Autodesk Inventor part; units mm, degrees
ref_plane "dia1_XY" through (-3.175, 3.9624, 0) normal (1, 0, 0) x (0, 0, -1)
ref_plane "dia1_YZ" through (-3.175, 3.9624, 0) normal (0, 0, -1) x (0, 1, 0)
ref_plane "dia1_ZX" through (-3.175, 3.9624, 0) normal (0, 1, 0) x (1, 0, 0)
sketch "Sketch_1" plane through (0, 0, 0) normal (0, 0, 1) x (1, 0, 0)
  line L0 (164.973, 0) -> (-3.175, 0)
  line L1 (-3.175, 0) -> (-3.175, 3.9624)
  line L2 (-3.175, 3.9624) -> (142.875, 3.9624)
  line L3 (142.875, 3.9624) -> (142.875, 13.5572)
  line L4 (142.875, 13.5572) -> (164.973, 13.5572)
  line L5 (164.973, 13.5572) -> (164.973, 0)
  line L6 (164.973, 0) -> (-3.175, 0)
revolve "Revolution1" add sketch "Sketch_1" angle 360 about axis through (164.973, 0, 0) along (1, 0, 0)
sketch "Sketch_3" plane through (0, 0, 0) normal (0, 0, 1) x (1, 0, 0)
  line L0 (-3.175, 0) -> (-15.875, 0)
  line L1 (-15.875, 0) -> (-15.875, 3.3388)
  line L2 (-15.875, 3.3388) -> (-15.2451, 3.9688)
  line L3 (-15.2451, 3.9688) -> (-3.175, 3.9688)
  line L4 (-3.175, 3.9688) -> (-3.175, 0)
  line L5 (-3.175, 0) -> (-15.875, 0)
revolve "Revolution2" add sketch "Sketch_3" angle 360 about axis through (-3.175, 0, 0) along (1, 0, 0)
thread "Thread1"
sketch "Sketch_10" plane through (-3.175, 0, 0) normal (1, 0, 0) x (0, 0, -1)
  line L0 (-7.9248, -7.9248) -> (7.9248, -7.9248)
  line L1 (7.9248, -7.9248) -> (7.9248, 7.9248)
  line L2 (7.9248, 7.9248) -> (-7.9248, 7.9248)
  line L3 (-7.9248, 7.9248) -> (-7.9248, -7.9248)
  line L4 (-3.175, -3.9624) -> (3.175, -3.9624)
  line L5 (3.175, -3.9624) -> (3.175, 3.9624)
  line L6 (3.175, 3.9624) -> (-3.175, 3.9624)
  line L7 (-3.175, 3.9624) -> (-3.175, -3.9624)
extrude "Extrusion1" cut sketch "Sketch_10" along normal blind 3.175
ref_plane "dia1_XY" through (-3.175, 3.9624, 0) normal (1, 0, 0) x (0, 0, -1)
ref_plane "dia1_YZ" through (-3.175, 3.9624, 0) normal (0, 0, -1) x (0, 1, 0)
ref_plane "dia1_ZX" through (-3.175, 3.9624, 0) normal (0, 1, 0) x (1, 0, 0)
ref_plane "dia12_XY" through (0, 0, 14.1351) normal (1, 0, 0) x (0, 0, -1)
ref_plane "dia12_YZ" through (0, 0, 14.1351) normal (0, 0, -1) x (0, 1, 0)
ref_plane "dia12_ZX" through (0, 0, 14.1351) normal (0, 1, 0) x (1, 0, 0)
ref_plane "dia2_XY" through (-3.175, -3.9624, 0) normal (1, 0, 0) x (0, 0, -1)
ref_plane "dia2_YZ" through (-3.175, -3.9624, 0) normal (0, 0, -1) x (0, 1, 0)
ref_plane "dia2_ZX" through (-3.175, -3.9624, 0) normal (0, 1, 0) x (1, 0, 0)
ref_plane "dia22_XY" through (0, 0, -14.1351) normal (1, 0, 0) x (0, 0, -1)
ref_plane "dia22_YZ" through (0, 0, -14.1351) normal (0, 0, -1) x (0, 1, 0)
ref_plane "dia22_ZX" through (0, 0, -14.1351) normal (0, 1, 0) x (1, 0, 0)
ref_plane "rl1_XY" through (-15.875, 0, 0) normal (1, 0, 0) x (0, 0, -1)
ref_plane "rl1_YZ" through (-15.875, 0, 0) normal (0, 0, -1) x (0, 1, 0)
ref_plane "rl1_ZX" through (-15.875, 0, 0) normal (0, 1, 0) x (1, 0, 0)
ref_plane "rl2_XY" through (-3.175, 0, 0) normal (1, 0, 0) x (0, 0, -1)
ref_plane "rl2_YZ" through (-3.175, 0, 0) normal (0, 0, -1) x (0, 1, 0)
ref_plane "rl2_ZX" through (-3.175, 0, 0) normal (0, 1, 0) x (1, 0, 0)
ref_plane "rod_cp_XY" through (0, 0, 0) normal (1, 0, 0) x (0, 0, -1)
ref_plane "rod_cp_YZ" through (0, 0, 0) normal (0, 0, -1) x (0, 1, 0)
ref_plane "rod_cp_ZX" through (0, 0, 0) normal (0, 1, 0) x (1, 0, 0)
ref_plane "thd1_XY" through (-15.875, 3.9688, 0) normal (1, 0, 0) x (0, 0, -1)
ref_plane "thd1_YZ" through (-15.875, 3.9688, 0) normal (0, 0, -1) x (0, 1, 0)
ref_plane "thd1_ZX" through (-15.875, 3.9688, 0) normal (0, 1, 0) x (1, 0, 0)
ref_plane "thd2_XY" through (-15.875, -3.9688, 0) normal (1, 0, 0) x (0, 0, -1)
ref_plane "thd2_YZ" through (-15.875, -3.9688, 0) normal (0, 0, -1) x (0, 1, 0)
ref_plane "thd2_ZX" through (-15.875, -3.9688, 0) normal (0, 1, 0) x (1, 0, 0)
ref_plane "to_rod_clevis_XY" through (-20.701, 0, 0) normal (1, 0, 0) x (0, 0, -1)
ref_plane "to_rod_clevis_YZ" through (-20.701, 0, 0) normal (0, 0, -1) x (0, 1, 0)
ref_plane "to_rod_clevis_ZX" through (-20.701, 0, 0) normal (0, 1, 0) x (1, 0, 0)
ref_plane "wf1_XY" through (-3.175, 0, 0) normal (1, 0, 0) x (0, 0, -1)
ref_plane "wf1_YZ" through (-3.175, 0, 0) normal (0, 0, -1) x (0, 1, 0)
ref_plane "wf1_ZX" through (-3.175, 0, 0) normal (0, 1, 0) x (1, 0, 0)
ref_plane "wf2_XY" through (0, 0, 0) normal (1, 0, 0) x (0, 0, -1)
ref_plane "wf2_YZ" through (0, 0, 0) normal (0, 0, -1) x (0, 1, 0)
ref_plane "wf2_ZX" through (0, 0, 0) normal (0, 1, 0) x (1, 0, 0)
ref_plane "wfw1_XY" through (-3.175, 0, -3.175) normal (0, 1, 0) x (1, 0, 0)
ref_plane "wfw1_YZ" through (-3.175, 0, -3.175) normal (1, 0, 0) x (0, 0, -1)
ref_plane "wfw1_ZX" through (-3.175, 0, -3.175) normal (0, 0, -1) x (0, 1, 0)
ref_plane "wfw2_XY" through (-3.175, 0, 3.175) normal (0, 1, 0) x (1, 0, 0)
ref_plane "wfw2_YZ" through (-3.175, 0, 3.175) normal (1, 0, 0) x (0, 0, -1)
ref_plane "wfw2_ZX" through (-3.175, 0, 3.175) normal (0, 0, -1) x (0, 1, 0)
properties part number "SR-094-D0_rod"
The model under review builds one solid part; all positions refer to its coordinate system, in mm. A direction names the side the tool comes from. Give positions to 0.01 mm unless a question says otherwise; leave off trailing zeros. Write each loop counter-clockwise with the first axis right and the second up, starting at its lowest first coordinate (ties: lowest second). Pieces come first, ordered by that corner, then holes. Notation, with made-up numbers: (0, 16.25) - (59, 16.25) arc R22 cw to (59, 29.25) - close; hole circle Ø2 at (23.5, -31.75). An arc over 180 degrees is marked (long way). Answer in a Markdown table with one row per item. Add a question column.
1. We need section A-A on z = 0. Write out the cut boundary in (x, y) (3 decimals).
2. We need section D-D on y = 9.75. Write out the cut boundary in (x, z) (3 decimals).
3. Tool access review of faces 5 (the flat face through (164.973, 0, 0)), 6 (the cylindrical face through (-9.126, 3.666, -1.52)): name each direction out of +Z, -Z, +X, -X, +Y, -Y from which nothing blocks a thin tool from reaching the whole face with its end or side.
4. Wall thickness on line 1 along X through (y, z) = (-0.5, -4.5) (3 decimals); line 2 along Z through (x, y) = (5, 0.25); line 3 along X through (y, z) = (3, -1.75): over which ranges is each line inside the solid? List them lowest first. Write a range as [from, to].
5. We need section C-C on x = 27. Write out the cut boundary in (y, z).
6. Draft analysis for pull direction X (two halves, no side actions). For faces 1 (the flat face through (-15.875, 0, 0)), 2 (the flat face through (-2, 0, -3.175)), 3 (the flat face through (-2, 0, 3.175)), 4 (the cylindrical face through (154.08, 12.93, 4.07)), state which applies: +X half, -X half, draft (parallel to the pull), parting line (faces both ways), or undercut.
7. Insertion check: P1, Ø2.5, axis at x = -2, y = 0.5, coming from the -Z side; P2, Ø5, axis at y = 10.5, z = -10.5, coming from the -X side (3 decimals); P3, Ø3.5, axis at x = -1, y = -0.5, coming from the +Z side. Each pin has a flat end and moves straight along its axis. Give the tip position at first contact, or say it passes through.
8. We need section B-B on y = 0. Write out the cut boundary in (x, z) (3 decimals), then the cut area to 3 significant figures.
Ans:
| question | item | result |
|---|---|---|
| 1 | outline | (-15.875, -3.339) - (-15.245, -3.969) - (-3.175, -3.969) - (-3.175, -3.962) - (142.875, -3.962) - (142.875, -13.557) - (164.973, -13.557) - (164.973, 13.557) - (142.875, 13.557) - (142.875, 3.962) - (-3.175, 3.962) - (-3.175, 3.969) - (-15.245, 3.969) - (-15.875, 3.339) - close |
| 2 | outline | (142.875, -9.42) - (164.973, -9.42) - (164.973, 9.42) - (142.875, 9.42) - close |
| 3 | face 5 | +Z, -Z, +X, +Y, -Y |
| 3 | face 6 | -X |
| 4 | line 1 | x = [142.875, 164.973] |
| 4 | line 2 | z = [-3.95, 3.95] |
| 4 | line 3 | x = [-15.74, 164.97] |
| 5 | outline | circle Ø7.92 at (0, 0) |
| 6 | face 1 | -X half |
| 6 | face 2 | undercut |
| 6 | face 3 | undercut |
| 6 | face 4 | draft |
| 7 | P1 | stops at z = -3.97 |
| 7 | P2 | stops at x = 142.875 |
| 7 | P3 | stops at z = 3.96 |
| 8 | outline | (-15.875, -3.339) - (-15.245, -3.969) - (-3.175, -3.969) - (-3.175, -3.175) - (0, -3.175) - (0, -3.962) - (142.875, -3.962) - (142.875, -13.557) - (164.973, -13.557) - (164.973, 13.557) - (142.875, 13.557) - (142.875, 3.962) - (0, 3.962) - (0, 3.175) - (-3.175, 3.175) - (-3.175, 3.969) - (-15.245, 3.969) - (-15.875, 3.339) - close |
| 8 | area | 1,850 mm^2 |
